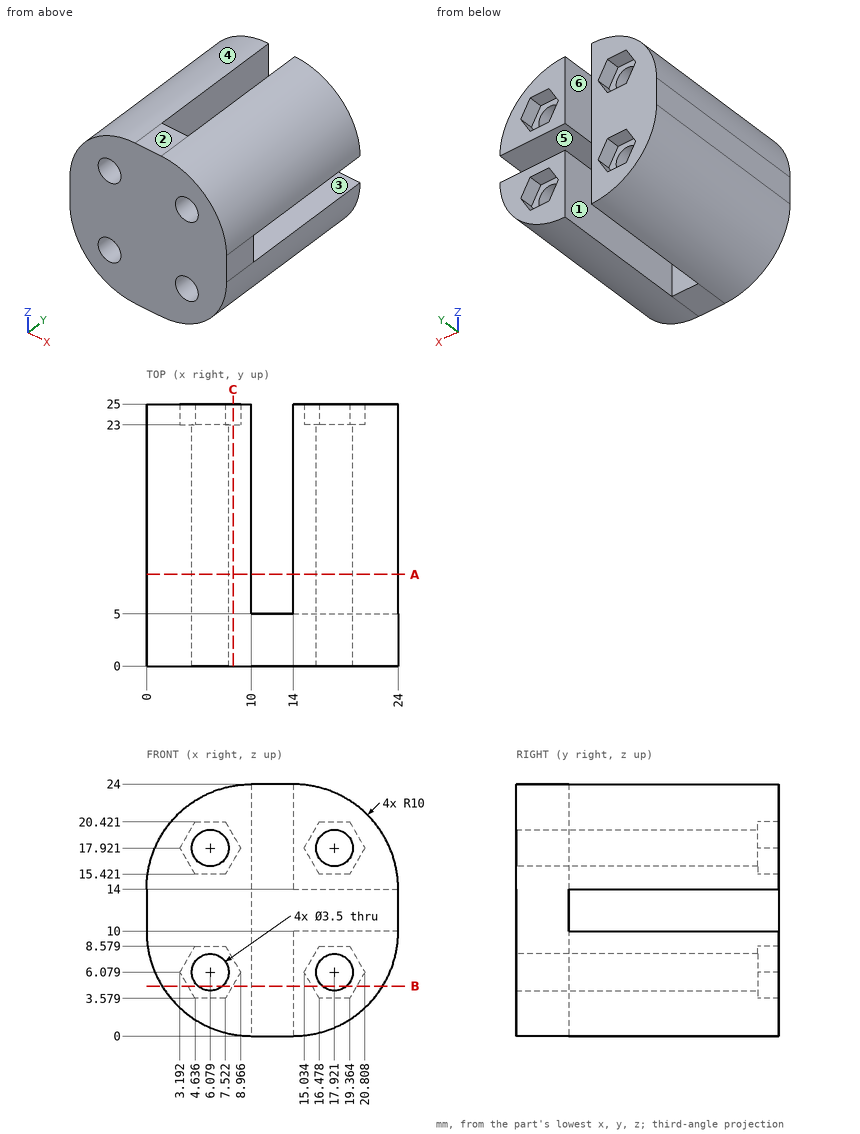
Here's the drawing with two shaded views (mm, measured from the low corner). I have some questions. A direction names the side the tool comes from. Give positions to 0.01 mm unless a question says otherwise; leave off trailing zeros. Order: outer loops, then holes, each group sorted by start corner. A loop starts at its lowest first (then second) coordinate and runs counter-clockwise, first axis right, second up. Notation, with made-up numbers: M 7,27.5 L 26,27.5 A5 cw 26,33.5 Z; hole C 12,-19 d3. An arc over 180 degrees is marked long. One line per item, written item: value.
1) I want a section at B-B, the plane z = 4.75. List the corners of the cut face in (x, y) for me.
Answer sheet:
outline: M 1.49,0 L 4.94,0 L 4.94,23 L 3.96,23 L 3.96,25 L 1.49,25 Z; M 7.22,0 L 16.78,0 L 16.78,23 L 15.8,23 L 15.8,25 L 14,25 L 14,5 L 10,5 L 10,25 L 8.2,25 L 8.2,23 L 7.22,23 Z; M 19.06,0 L 22.51,0 L 22.51,25 L 20.04,25 L 20.04,23 L 19.06,23 Z
2) We'd pull the mould along Z, two halves only. Please class the marked faces 1, 2 and 3: released by +Z, released by -Z, zero draft, split by the parting line, or undercut.
Answer sheet:
face 1: zero draft
face 2: released by +Z
face 3: undercut
3) For P1, Ø1, axis at y = 22, z = 18.5, coming from the +X side (1 decimal); P2, Ø6, axis at x = 21.5, y = 15.5, coming from the -Z side; P3, Ø0.6, axis at x = 6, y = 24, coming from the +Z side, each with a flat end and sliding along its axis, tell me the tip position at first contact or that it passes through.
Answer sheet:
P1: stops at x = 23.2
P2: stops at z = 1.07
P3: stops at z = 23.29
4) I want a section at C-C, the plane x = 8.25. List the corners of the cut face in (y, z) for me (1 decimal).
Answer sheet:
outline: M 0,0.2 L 25,0.2 L 25,4.8 L 23,4.8 L 23,7.3 L 25,7.3 L 25,16.7 L 23,16.7 L 23,19.2 L 25,19.2 L 25,23.8 L 0,23.8 Z
5) On a 3-axis mill with a long thin cutter (end or side, diameter ignored), from which of +Z, -Z, +X, -X, +Y, -Y can I reach the whole of each face in a straight line? I mean the marked faces 4, 5 and 6. Say none if no direction works.
Answer sheet:
face 4: +Z, -X, +Y, -Y
face 5: +X, +Y
face 6: +Z, -Z, +Y
6) Please list where these lines run through material, in increasing order: line 1 along X through (y, z) = (18.5, 7) (1 decimal); line 2 along Z through (x, y) = (7, 12.5) (1 decimal); line 3 along Z through (x, y) = (7.5, 7.25) (1 decimal).
Answer sheet:
line 1: x = 0.5 to 4.6, 7.6 to 10, 14 to 16.4, 19.4 to 23.5
line 2: z = 0.5 to 4.6, 7.6 to 16.4, 19.4 to 23.5
line 3: z = 0.3 to 5.1, 7.1 to 16.9, 18.9 to 23.7
7) I want a section at A-A, the plane y = 8.75. Count the separate pieces of the cut face and the enclosed holes in it, plus the area to 3 significant figures.
Answer sheet:
separate pieces: 3
enclosed holes: 4
area: 316 mm^2
